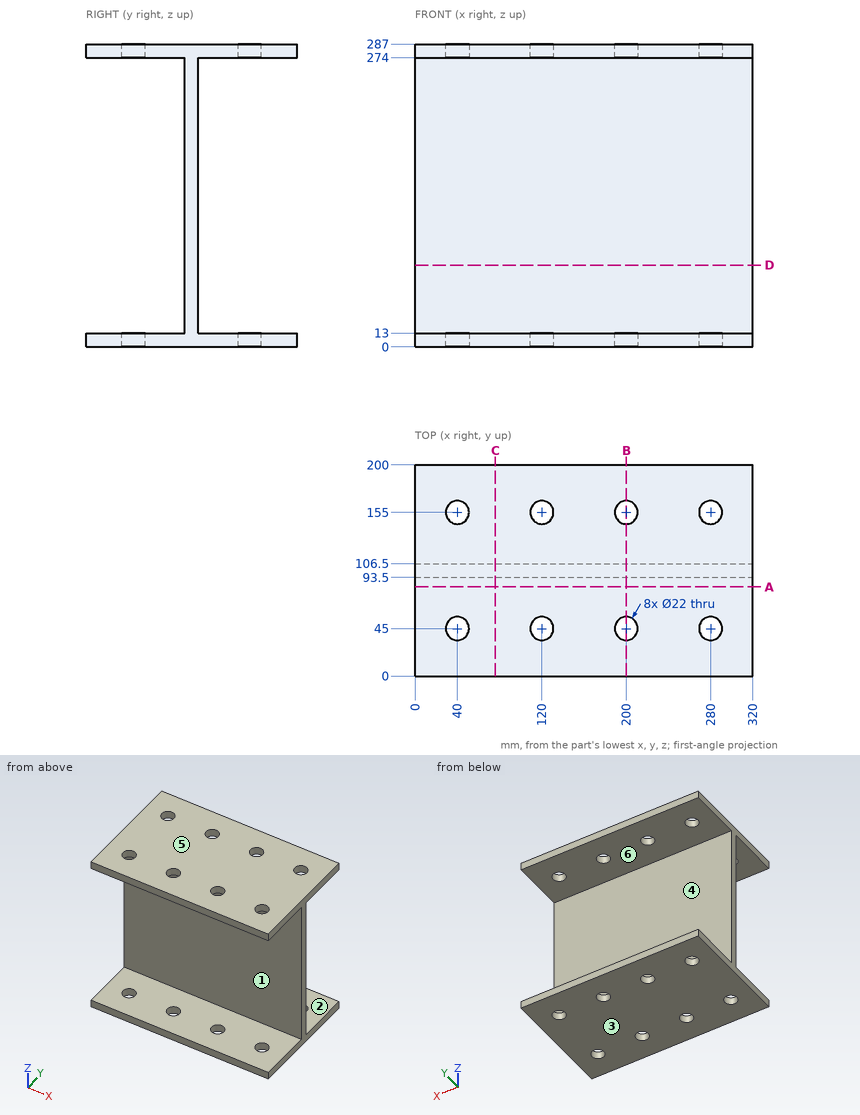
Part print with two shaded views. Sizes in mm from the minimum x, y, z corner. A direction names the side the tool comes from. Round coordinates to 2 decimals unless told otherwise and drop trailing zeros. Order: outer loops, then holes, each group sorted by start corner. A loop starts at its lowest first (then second) coordinate and runs counter-clockwise, first axis right, second up. Notation, with made-up numbers: M 34,22 L 81,22 A17 cw 81,42 Z; hole C -7,73 d1. An arc over 180 degrees is marked long. Put each result on its own line as item: value. Start each with the question number.
1. Slice it at A-A on y = 84.5. List the corners of the cut face in (x, z).
2. Slice it at D-D on z = 77.5. List the corners of the cut face in (x, y).
3. Slice it at B-B on x = 200. List the corners of the cut face in (y, z).
4. Tool access for the marked faces 1 and 2: list every direction of +Z, -Z, +X, -X, +Y, -Y with a clear straight run to the whole face (end or side of a thin tool).
5. Slice it at C-C on x = 76. List the corners of the cut face in (y, z), then the cut area to 3 significant figures.
6. Drill centre lines: probe 1 along Y at (x, z) = (120, 278); probe 2 along Z at (x, y) = (95.5, 141); probe 3 along Y at (x, z) = (264, 104). Where is each one in solid material? Low to high. Write a range as [from, to].
7. Drop flat-ended pins along their axis: pin 1 (10 mm diameter, centred on x = 273.5, z = 141, fed in from -Y); pin 2 (2 mm diameter, centred on x = 159.5, z = 51, fed in from +Y). Give the stop position or say it passes through.
8. Two-plate mould, pull along Z, no slides. Class the marked faces 3, 4, 5 and 6: +Z half, -Z half, draft (parallel to the pull), parting line (faces both ways), or undercut.
Findings:
1. outline: M 0,0 L 320,0 L 320,13 L 0,13 Z; M 0,274 L 320,274 L 320,287 L 0,287 Z
2. outline: M 0,93.5 L 320,93.5 L 320,106.5 L 0,106.5 Z
3. outline: M 0,0 L 34,0 L 34,13 L 0,13 Z; M 0,274 L 34,274 L 34,287 L 0,287 Z; M 56,0 L 144,0 L 144,13 L 106.5,13 L 106.5,274 L 144,274 L 144,287 L 56,287 L 56,274 L 93.5,274 L 93.5,13 L 56,13 Z; M 166,0 L 200,0 L 200,13 L 166,13 Z; M 166,274 L 200,274 L 200,287 L 166,287 Z
4. face 1: +X, -X, -Y
4. face 2: +X, -X, +Y
5. outline: M 0,0 L 200,0 L 200,13 L 106.5,13 L 106.5,274 L 200,274 L 200,287 L 0,287 L 0,274 L 93.5,274 L 93.5,13 L 0,13 Z
5. area: 8,590 mm2
6. probe 1: [0, 34], [56, 144], [166, 200]
6. probe 2: [0, 13], [274, 287]
6. probe 3: [93.5, 106.5]
7. pin 1: y = 93.5
7. pin 2: y = 106.5
8. face 3: -Z half
8. face 4: undercut
8. face 5: +Z half
8. face 6: undercut
